Geometry check sheet. Reference: the model listing, model coordinates, mm. Face numbers are marked on the shaded views. A direction names the side the tool comes from. Round coordinates to 2 decimals unless told otherwise and drop trailing zeros. Order: outer loops, then holes, each group sorted by start corner. A loop starts at its lowest first (then second) coordinate and runs counter-clockwise, first axis right, second up. Notation, with made-up numbers: (35, -1) - (72, -1) arc R21 ccw to (72, 33) - close; hole circle Ø2 at (-37.75, 21). An arc over 180 degrees is marked (long way). One line per question, with ' | ' between items. Start each with the question number.
Q1. Material ranges on line 1 along X through (y, z) = (-28.5, 10); line 2 along Z through (x, y) = (46, 14); line 3 along X through (y, z) = (-22, 18), recorded low to high.
Q2. Gauge pin test, flat ends, axial feed: P1, Ø2, axis at x = 22.5, z = 2.5, coming from the +Y side; P2, Ø1.6, axis at x = 40, z = 10, coming from the +Y side; P3, Ø10, axis at y = -21, z = 2.5, coming from the +X side. Record the tip position at first contact, or that the pin passes through.
Q3. Tool access check on the marked faces 1, 2, 3, 4 and 5. Record the directions out of +Z, -Z, +X, -X, +Y, -Y that give a thin tool (end or side, any length) a straight path to the whole face; none if there is none.
Q4. Sectioned sample at B-B, the plane y = -3. Enter the section's corners in (x, z).
Q5. Sectioned sample at A-A, the plane z = 10. Enter the section's corners in (x, y), then the cut area to 3 significant figures.
Q6. Sectioned sample at D-D, the plane y = 18.5. Enter the section's corners in (x, z), then the cut area to 3 significant figures.
Q7. Mould release check, pull along X, two halves, no side actions. Record for the marked faces 6, 7 and 8: +X half, -X half, draft (parallel to the pull), parting line (faces both ways), or undercut.
Q8. Sectioned sample at C-C, the plane z = 2. Enter the section's corners in (x, y), then the cut area to 3 significant figures.
```python
from build123d import *

# Parameters (mm, degrees)
SZKIC1_R                    = 4
DODANIE_WYCI_GNI_CIE1_DEPTH = 20
SZKIC2_W                    = 28.4
SZKIC2_H                    = 10
WYTNIJ_WYCI_GNI_CIE1_DEPTH  = 22
SZKIC3_R                    = 3
WYTNIJ_WYCI_GNI_CIE2_DEPTH  = 89.667893976
SZKIC4_R                    = 6
WYTNIJ_WYCI_GNI_CIE3_DEPTH  = 54.5
WYTNIJ_WYCI_GNI_CIE5_DEPTH  = 74.489764063
ZAOKR_GLENIE1_R             = 10
WYTNIJ_WYCI_GNI_CIE6_DEPTH  = 74.489764063
ZAOKR_GLENIE2_R             = 7
ZAOKR_GLENIE3_R             = 4
ZAOKR_GLENIE4_R             = 0.4
ZAOKR_GLENIE5_R             = 0.2


with BuildPart() as part:
    # Szkic1 → Dodanie-wyciągnięcie1 (new body)
    with BuildSketch(Plane.XY):
        Polygon((15.55899167, -31), (63.55899167, -31), (63.55899167, -27), (48.75899167, 4.5), (48.75899167, 27.5), (30.35899167, 27.5), (30.35899167, 4.5), (15.55899167, -27), align=None)
        with Locations((39.55899167, 18.5)):
            Circle(SZKIC1_R, mode=Mode.SUBTRACT)
    extrude(amount=DODANIE_WYCI_GNI_CIE1_DEPTH)

    # Szkic2 → Wytnij-wyciągnięcie1 (cut)
    with BuildSketch(Plane(origin=(0, 27.5, 0), x_dir=(1, 0, 0), z_dir=(0, 1, 0))):
        with Locations((39.55899167, -10)):
            Rectangle(SZKIC2_W, SZKIC2_H)
    extrude(amount=-WYTNIJ_WYCI_GNI_CIE1_DEPTH, mode=Mode.SUBTRACT)

    # Szkic3 → Wytnij-wyciągnięcie2 (cut, through all)
    with BuildSketch(Plane(origin=(0, 27.5, 0), x_dir=(1, 0, 0), z_dir=(0, 1, 0))):
        with Locations(Location((56.55899167, -10, 0), (0, 0, 270))):
            Circle(SZKIC3_R)
        with Locations(Location((22.55899167, -10, 0), (0, 0, 270))):
            Circle(SZKIC3_R)
    extrude(amount=-WYTNIJ_WYCI_GNI_CIE2_DEPTH, mode=Mode.SUBTRACT)

    # Szkic4 → Wytnij-wyciągnięcie3 (cut)
    with BuildSketch(Plane(origin=(0, 27.5, 0), x_dir=(1, 0, 0), z_dir=(0, 1, 0))):
        with Locations(Location((56.55899167, -10, 0), (0, 0, 270))):
            Circle(SZKIC4_R)
        with Locations(Location((22.55899167, -10, 0), (0, 0, 270))):
            Circle(SZKIC4_R)
    extrude(amount=-WYTNIJ_WYCI_GNI_CIE3_DEPTH, mode=Mode.SUBTRACT)

    # Szkic6 → Wytnij-wyciągnięcie5 (cut, through all)
    with BuildSketch(Plane(origin=(0, 0, 0), x_dir=(-1, 0, 0), z_dir=(0, 0, -1))):
        with BuildLine():
            Line((-63.55899167, -27), (-55.55899167, -27))
            Line((-55.55899167, -27), (-45.422866973, 19.770813293))
            ThreePointArc((-45.422866973, 19.770813293), (-39.55899167, 24.5), (-33.695116367, 19.770813293))
            Line((-33.695116367, 19.770813293), (-23.55899167, -27))
            Line((-23.55899167, -27), (-15.55899167, -27))
            Line((-15.55899167, -27), (-15.55899167, 33))
            Line((-15.55899167, 33), (-63.55899167, 33))
            Line((-63.55899167, 33), (-63.55899167, -27))
        make_face()
    extrude(amount=-WYTNIJ_WYCI_GNI_CIE5_DEPTH, mode=Mode.SUBTRACT)

    # Zaokrąglenie1
    # the kernel refuses this fillet: 10 mm, written as the material it takes off along each edge
    with BuildSketch(Plane(origin=(63.55899167, -56, 20), x_dir=(0, 0, -1), z_dir=(0, 1, 0)), Plane(origin=(15.55899167, -2, 0), x_dir=(1, 0, 0), z_dir=(0, -1, 0))) as zaokr_glenie1_piece_1:
        with BuildLine():
            CenterArc((ZAOKR_GLENIE1_R, ZAOKR_GLENIE1_R), ZAOKR_GLENIE1_R, 180, 90)
            Line((0, ZAOKR_GLENIE1_R), (0, 0))
            Line((0, 0), (ZAOKR_GLENIE1_R, 0))
        make_face()
    extrude(amount=54, mode=Mode.SUBTRACT)
    with BuildSketch(Plane(origin=(63.55899167, -56, 0), x_dir=(0, 0, 1), z_dir=(0, 1, 0)), Plane(origin=(15.55899167, -2, 20), x_dir=(1, 0, 0), z_dir=(0, -1, 0))) as zaokr_glenie1_piece_2:
        with BuildLine():
            CenterArc((ZAOKR_GLENIE1_R, -ZAOKR_GLENIE1_R), ZAOKR_GLENIE1_R, 90, 90)
            Line((0, -ZAOKR_GLENIE1_R), (0, 0))
            Line((0, 0), (ZAOKR_GLENIE1_R, 0))
        make_face()
    extrude(amount=54, mode=Mode.SUBTRACT)

    # Szkic7 → Wytnij-wyciągnięcie6 (cut, through all)
    with BuildSketch(Plane(origin=(0, 0, 0), x_dir=(-1, 0, 0), z_dir=(0, 0, -1))):
        with BuildLine():
            Line((-46.400179524, -18.517384491), (-42.490929322, -0.479049644))
            ThreePointArc((-42.490929322, -0.479049644), (-39.55899167, 1.885543709), (-36.627054018, -0.479049644))
            Line((-36.627054018, -0.479049644), (-32.717803816, -18.517384491))
            ThreePointArc((-32.717803816, -18.517384491), (-39.55899167, -27), (-46.400179524, -18.517384491))
        make_face()
    extrude(amount=-WYTNIJ_WYCI_GNI_CIE6_DEPTH, mode=Mode.SUBTRACT)

    # Zaokrąglenie2
    zaokr_glenie2_edges = [part.edges().sort_by_distance(p)[0] for p in [
        (55.55899167, -27, 17.857019377),
        (55.55899167, -27, 2.142980623),
        (23.55899167, -27, 17.857019377),
        (23.55899167, -27, 2.142980623),
    ]]
    fillet(zaokr_glenie2_edges, radius=ZAOKR_GLENIE2_R)

    # Zaokrąglenie3
    zaokr_glenie3_edges = [part.edges().sort_by_distance(p)[0] for p in [
        (39.55899167, 5.5, 5),
        (39.55899167, 5.5, 15),
    ]]
    fillet(zaokr_glenie3_edges, radius=ZAOKR_GLENIE3_R)

    # Zaokrąglenie4
    zaokr_glenie4_edges = [part.edges().sort_by_distance(p)[0] for p in [
        (50.55899167, -27, 10),
        (28.55899167, -27, 10),
    ]]
    fillet(zaokr_glenie4_edges, radius=ZAOKR_GLENIE4_R)

    # Zaokrąglenie5
    zaokr_glenie5_edges = [part.edges().sort_by_distance(p)[0] for p in [
        (35.55899167, 18.5, 0),
        (35.55899167, 18.5, 20),
        (35.55899167, 18.5, 15),
    ]]
    fillet(zaokr_glenie5_edges, radius=ZAOKR_GLENIE5_R)


solid = part.part
```
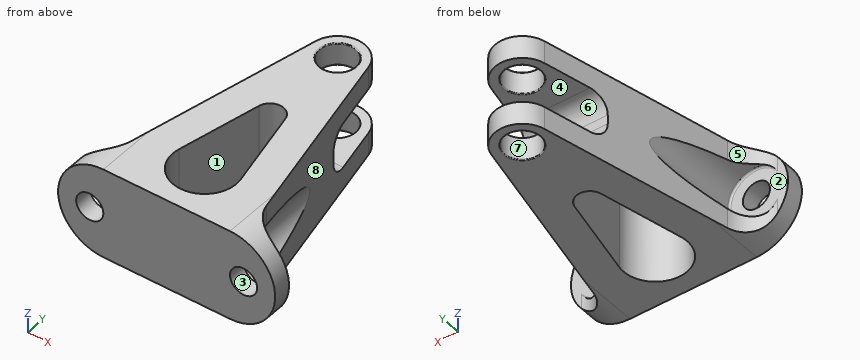
Determined:
1) line 1: x = 15.56 to 19.56, 25.56 to 53.56, 59.56 to 63.56 | line 2: z = 0 to 5, 15 to 20 | line 3: x = 24.62 to 32.85, 46.27 to 54.5
2) P1: stops at y = -24.22 | P2: stops at y = 5.5 | P3: stops at x = 57.6
3) face 1: +Z, -Z | face 2: +Y | face 3: +Y, -Y | face 4: +X, -X, +Y | face 5: +Z, -Z, -X, +Y
4) outline: (28.76, 0) - (36.08, 0) - (36.08, 20) - (28.76, 20) - close; (43.04, 0) - (50.36, 0) - (50.36, 20) - (43.04, 20) - close
5) outline: (15.56, -31) - (19.56, -31) - (19.56, -27) - (15.56, -27) - close; (25.56, -31) - (53.56, -31) - (53.56, -27) - (50.96, -27) arc R0.4 cw to (50.56, -26.6) - (50.56, -3.93) - (48.52, 5.5) - (30.6, 5.5) - (28.56, -3.93) - (28.56, -26.6) arc R0.4 cw to (28.16, -27) - (25.56, -27) - close; (59.56, -31) - (63.56, -31) - (63.56, -27) - (59.56, -27) - close; hole (32.72, -18.52) arc R7 ccw (long way) to (46.4, -18.52) - (42.49, -0.48) arc R3 ccw to (36.63, -0.48) - close | area: 556 mm2
6) outline: (33.42, 0) - (35.36, 0) arc R0.2 ccw to (35.56, 0.2) - (35.56, 5) - (33.42, 5) - close; (33.42, 15) - (35.36, 15) arc R0.2 ccw to (35.56, 15.2) - (35.56, 19.8) arc R0.2 ccw to (35.36, 20) - (33.42, 20) - close; (43.56, 0.2) arc R0.2 ccw to (43.76, 0) - (45.7, 0) - (45.7, 5) - (43.56, 5) - close; (43.56, 15.2) arc R0.2 ccw to (43.76, 15) - (45.7, 15) - (45.7, 20) - (43.76, 20) arc R0.2 ccw to (43.56, 19.8) - close | area: 42.7 mm2
7) face 6: draft | face 7: undercut | face 8: +X half
8) outline: (19.56, -31) - (59.56, -31) - (59.56, -26.8) arc R7 cw to (54.36, -21.48) - (45.42, 19.77) arc R6 ccw to (33.7, 19.77) - (24.75, -21.48) arc R7 cw to (19.56, -26.8) - close; hole (32.72, -18.52) arc R7 ccw (long way) to (46.4, -18.52) - (42.49, -0.48) arc R3 ccw to (36.63, -0.48) - close; hole circle Ø8 at (39.56, 18.5) | area: 902 mm2
